Model file for the job. Use its own axes, mm. Face numbers are marked on the shaded views. Round coordinates to 2 decimals unless told otherwise and drop trailing zeros. Write each loop counter-clockwise with the first axis right and the second up, starting at its lowest first coordinate (ties: lowest second). Pieces come first, ordered by that corner, then holes. Notation, with made-up numbers: (7.5, 88) - (11.5, 88) arc R32 cw to (11.5, 125) - close; hole circle Ø1 at (23.5, 52). An arc over 180 degrees is marked (long way). One line per item, written item: value.
from build123d import *

# Parameters (mm, degrees)
F0_W      = 0.3302
F0_H      = 107.95
F2_R      = 3.175
F3_DEPTH  = 12.3962
F6_R      = 3.175
F7_DEPTH  = 1.7554578348
F10_DEPTH = 1.7554578348


with BuildPart() as f1:
    # F0 (on Front) → F1 (revolve)
    with BuildSketch(Plane.XZ):
        with Locations((12.2301, 53.975)):
            Rectangle(F0_W, F0_H)
    revolve(axis=Axis((0, 0, 53.975), (0, 0, 1)))

    # F2 (on Front) → F3 (cut, through all)
    with BuildSketch(Plane.XZ):
        with Locations((0, 82.55)):
            Circle(F2_R)
    extrude(amount=F3_DEPTH, mode=Mode.SUBTRACT)

    # F6 (on line) → F7 (cut, up to face)
    with BuildSketch(Plane(origin=(10.734558085, 6.1976, 0), x_dir=(-0.5, 0.8660254038, 0), z_dir=(0.8660254038, 0.5, 0))):
        with Locations((0, 82.55)):
            Circle(F6_R)
    extrude(amount=-F7_DEPTH, mode=Mode.SUBTRACT)

    # F9 (on line) → F10 (cut, up to face)
    with BuildSketch(Plane(origin=(-10.734558085, 6.1976, 0), x_dir=(-0.5, -0.8660254038, 0), z_dir=(-0.8660254038, 0.5, 0))):
        with BuildLine():
            ThreePointArc((0, 85.725), (-3.175, 82.55), (0, 79.375))
            Line((0, 79.375), (0, 85.725))
        make_face()
        with BuildLine():
            Line((0, 85.725), (0, 79.375))
            ThreePointArc((0, 79.375), (2.2450640303, 80.3049359697), (3.175, 82.55))
            ThreePointArc((3.175, 82.55), (2.2450640303, 84.7950640303), (0, 85.725))
        make_face()
    extrude(amount=-F10_DEPTH, mode=Mode.SUBTRACT)


solid = f1.part
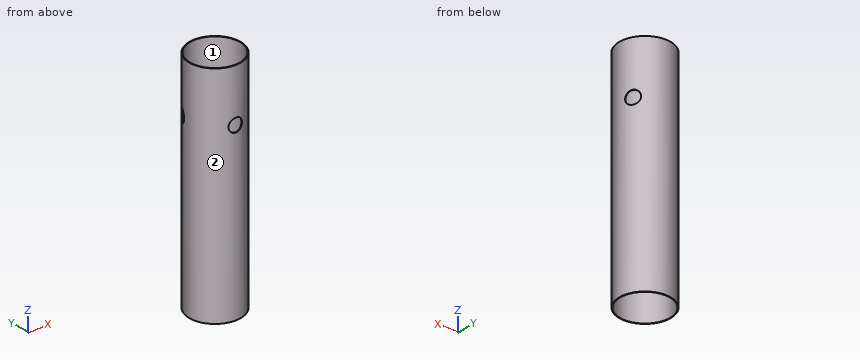
1. Wall check: probe 1 along Z at (x, y) = (0, -12.1) (3 decimals); probe 2 along Y at (x, z) = (0, 45.5) (3 decimals); probe 3 along X at (y, z) = (2.75, 31). Give the ranges that are in metal, low to high. Write a range as [from, to].
Report:
probe 1: [0, 79.375], [85.725, 107.95]
probe 2: [-12.395, -12.065], [12.065, 12.395]
probe 3: [-12.09, -11.75], [11.75, 12.09]
2. Band-saw the part on A-A on x = 0. Write the cut outline in (y, z) (3 decimals).
Report:
outline: (-12.395, 0) - (-12.065, 0) - (-12.065, 79.375) - (-12.395, 79.375) - close; (-12.395, 85.725) - (-12.065, 85.725) - (-12.065, 107.95) - (-12.395, 107.95) - close; (12.065, 0) - (12.395, 0) - (12.395, 107.95) - (12.065, 107.95) - close
3. Band-saw the part on C-C on z = 40. Write the cut outline in (x, y) (3 decimals), plus the area to 3 significant figures.
Report:
outline: circle Ø24.79 at (0, 0); hole circle Ø24.13 at (0, 0)
area: 25.4 mm²
4. Drop flat-ended pins along their axis: pin 1 (10 mm diameter, centred on x = 7, z = 46.5, fed in from -Y); pin 2 (6 mm diameter, centred on x = -5.5, y = -6, fed in from -Z); pin 3 (6 mm diameter, centred on y = 9.5, z = 77.5, fed in from +X); pin 4 (5 mm diameter, centred on x = 0, z = 82.55, fed in from -Y). Give the stop position or say it passes through.
Report:
pin 1: y = -12.23
pin 2: through
pin 3: x = 10.55
pin 4: y = 11.8
5. Band-saw the part on D-D on x = 5. Write the cut outline in (y, z).
Report:
outline: (-11.34, 0) - (-10.98, 0) - (-10.98, 107.95) - (-11.34, 107.95) - close; (10.98, 0) - (11.34, 0) - (11.34, 107.95) - (10.98, 107.95) - close
6. Mould opens along X. For the marked faces 1 and 2 say: released by +X, released by -X, zero draft, split by the parting line, or undercut.
Report:
face 1: undercut
face 2: split by the parting line
